Autodesk Inventor part; units mm, degrees
ref_plane "YZ Plane" through (0, 0, 0) normal (1, 0, 0) x (0, 1, 0)
ref_plane "XZ Plane" through (0, 0, 0) normal (0, 1, 0) x (-1, 0, 0)
ref_plane "XY Plane" through (0, 0, 0) normal (0, 0, 1) x (1, 0, 0)
sketch "Sketch1" plane through (0, 0, 0) normal (0, 0, 1) x (1, 0, 0)
  line L0 (0, 0) -> (12.7, 0)
  line L1 (12.7, 0) -> (12.7, -11.43)
  line L2 (6.35, -17.78) -> (6.35, -17.78)
  line L3 (0, -11.43) -> (0, 0)
  arc A0 (6.35, -17.78) -> (12.7, -11.43) centre (6.35, -11.43) ccw
  arc A1 (0, -11.43) -> (6.35, -17.78) centre (6.35, -11.43) ccw
  point P0 (12.7, -17.78)
  point P1 (0, -17.78)
  dimension "d0" = 12.7
  dimension "d1" = 17.78
  dimension "d2" = 6.35
extrude "Extrusion1" add sketch "Sketch1" along normal blind 3.175
sketch "Sketch2" plane through (0, 0, 3.175) normal (0, 0, 1) x (1, 0, 0)
  line L0 (12.7, 0) -> (0, 0)
  line L1 (0, 0) -> (0, -11.43)
  arc A0 (0, -11.43) -> (12.7, -11.43) centre (6.35, -11.43) ccw
  line L2 (12.7, -11.43) -> (12.7, 0)
  line L3 (-3.175, 3.175) -> (15.875, 3.175)
  line L4 (15.875, 3.175) -> (15.875, -11.43)
  arc A1 (-3.175, -11.43) -> (15.875, -11.43) centre (6.35, -11.43) ccw
  line L5 (-3.175, -11.43) -> (-3.175, 3.175)
  dimension "d5" = 3.175
extrude "Extrusion2" add sketch "Sketch2" against normal blind 6.223
sketch "Sketch3" plane through (0, 0, -3.048) normal (0, 0, -1) x (-1, 0, 0)
  line L0 (-15.875, 3.175) -> (-15.875, -11.43)
  line L1 (-15.875, 3.175) -> (3.351, 3.175)
  line L2 (3.351, 3.175) -> (3.351, 0)
  line L3 (3.351, 0) -> (-15.875, 0)
  line L4 (-15.875, 0) -> (-15.875, 3.175)
  line L5 (-12.7, 0) -> (0, 0)
  line L6 (3.175, 3.175) -> (-15.875, 3.175)
  line L7 (-12.7, 0) -> (0, 0)
  line L8 (0, 0) -> (0, 3.175)
  line L9 (0, 3.175) -> (-12.7, 3.175)
  line L10 (-12.7, 3.175) -> (-12.7, 0)
extrude "Extrusion3" cut sketch "Sketch3" against normal blind 3.048 contours L1 L8 L3 L10
sketch "Sketch4" plane through (0, 0, 0) normal (0, 0, -1) x (-1, 0, 0)
  arc A0 (-12.7, -11.43) -> (0, -11.43) centre (-6.35, -11.43) ccw
  circle A1 centre (-6.35, -11.43) radius 2.54
  point P0 (0, 0)
  dimension "d10" = 5.08
extrude "Extrusion4" cut sketch "Sketch4" against normal blind 25.4
properties part number "new jewel fail"
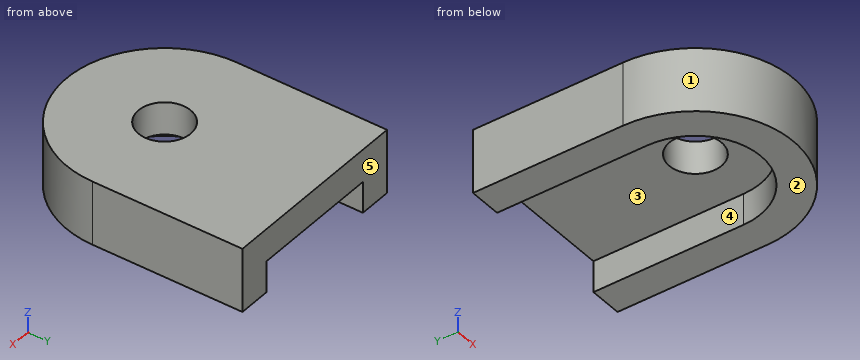
Can you work these out from the model? Positions are in its coordinate system, mm. Face numbers are marked on the shaded views. A direction names the side the tool comes from. Round coordinates to 2 decimals unless told otherwise and drop trailing zeros. Loops run counter-clockwise (first coordinate to the right, second up) from the corner with the lowest first, then second, coordinate; pieces in that order, holes last.
Item 1: Suppose I cut it at D-D, the plane x = 11.5. Write out the boundary of the cut face in (y, z) (3 decimals), then the cut area to 3 significant figures.
Item 2: Will these pins go through, and if not, where does the flat tip stop? pin 1 Ø4 at (x, y) = (3.5, -9) entering from -Z; pin 2 Ø6.5 at (x, y) = (6.35, -11.43) entering from +Z (3 decimals).
Item 3: Which directions (+Z, -Z, +X, -X, +Y, -Y) give clear straight access to the entire face, cutting with the end or side of a thin tool? Please do the marked faces 4 and 5.
Item 4: If we mould it in two halves opening along X, with no side actions, what happens to the marked faces 1, 2 and 3? For each: +X half, -X half, draft (parallel to the pull), parting line (faces both ways), or undercut.
Item 5: Please list where these lines run through material, in increasing order: L1, parallel to Y at x = 6.35, z = 1.25 (3 decimals); L2, parallel to X at y = 1.25, z = -1.5 (3 decimals); L3, parallel to Z at x = 9.5, y = -14.25 (3 decimals).
Item 6: Suppose I cut it at C-C, the plane z = -1.5. Write out the boundary of the cut face in (x, y) (3 decimals).
Item 7: Suppose I cut it at A-A, the plane x = 6.35. Write out the boundary of the cut face in (y, z) (3 decimals).
Item 8: Suppose I cut it at B-B, the plane z = 1.25. Write out the boundary of the cut face in (x, y) (3 decimals), then the cut area to 3 significant figures.
Reported:
1. outline: (-19.443, -3.048) - (-15.145, -3.048) - (-15.145, 0) - (3.175, 0) - (3.175, 3.175) - (-19.443, 3.175) - close
1. area: 84.9 mm2
2. pin 1: stops at z = 0
2. pin 2: stops at z = 3.175
3. face 4: -Z, +Y
3. face 5: +Z, -Z, +X, -X, +Y
4. face 1: parting line
4. face 2: draft
4. face 3: undercut
5. L1: y = -20.955 to -13.97, -8.89 to 3.175
5. L2: x = -3.175 to 0, 12.7 to 15.875
5. L3: z = 0 to 3.175
6. outline: (-3.175, -11.43) arc R9.525 ccw to (15.875, -11.43) - (15.875, 3.175) - (12.7, 3.175) - (12.7, -11.43) arc R6.35 cw to (0, -11.43) - (0, 3.175) - (-3.175, 3.175) - close
7. outline: (-20.955, -3.048) - (-17.78, -3.048) - (-17.78, 0) - (-13.97, 0) - (-13.97, 3.175) - (-20.955, 3.175) - close; (-8.89, 0) - (3.175, 0) - (3.175, 3.175) - (-8.89, 3.175) - close
8. outline: (-3.175, -11.43) arc R9.525 ccw to (15.875, -11.43) - (15.875, 3.175) - (-3.175, 3.175) - close; hole circle Ø5.08 at (6.35, -11.43)
8. area: 400 mm2
